```python
from build123d import *

# Parameters (mm, degrees)
F0_W     = 889
F0_H     = 762
F1_DEPTH = 1778
F2_W     = 25.4
F2_H     = 1778
F3_DEPTH = 50.8
F4_W     = 203.0948400497
F4_H     = 157.5736999512
F5_DEPTH = 50.8
F6_SIZE  = 12.7
F7_R     = 38.09999


# Not quite as in the source:
# - a fillet or chamfer is up to 0.001 mm smaller than in the source, because OpenCascade refuses the exact size


with BuildPart() as f1:
    # F0 (on Top) → F1 (new body)
    with BuildSketch(Plane.XY):
        with Locations((444.5, 381)):
            Rectangle(F0_W, F0_H)
    extrude(amount=F1_DEPTH)

    # F2 (on face) → F3 (cut)
    with BuildSketch(Plane.XZ):
        with Locations((431.8, 889)):
            Rectangle(F2_W, F2_H)
    extrude(amount=-F3_DEPTH, mode=Mode.SUBTRACT)

    # F4 (on face) → F5 (cut)
    with BuildSketch(Plane.XZ):
        with Locations((695.2850222588, 1232.5783967972)):
            Rectangle(F4_W, F4_H)
    extrude(amount=-F5_DEPTH, mode=Mode.SUBTRACT)

    # F6
    f6_edges = [f1.edges().sort_by_distance(p)[0] for p in [
        (695.285022, 50.8, 1311.365247),
        (593.737602, 50.8, 1232.578397),
        (695.285022, 50.8, 1153.791547),
        (796.832442, 50.8, 1232.578397),
    ]]
    chamfer(f6_edges, length=F6_SIZE)

    # F7 (radius 38.1 in the source; OpenCascade refuses exactly that, so slightly less here)
    f7_edges = [f1.edges().sort_by_distance(p)[0] for p in [
        (209.55, 0, 0),
        (419.1, 0, 889),
        (209.55, 0, 1778),
        (0, 0, 889),
        (666.75, 0, 0),
        (444.5, 0, 889),
        (889, 0, 889),
        (666.75, 0, 1778),
        (796.832442, 0, 1232.578397),
        (695.285022, 0, 1153.791547),
        (593.737602, 0, 1232.578397),
        (695.285022, 0, 1311.365247),
    ]]
    fillet(f7_edges, radius=F7_R)


solid = f1.part
```
Work out the finished part from the listing and answer in its coordinate system (mm). A direction names the side the tool comes from. Round coordinates to 2 decimals unless told otherwise and drop trailing zeros. Write each question's results on one line, items separated by ' | '.
Q1. Straight lines are drawn through the part: line 1 along X through (y, z) = (34, 98); line 2 along Y through (x, z) = (670.5, 1284.5); line 3 along Z through (x, y) = (397, 36.5). For each, find the intervals that lie inside material, in ascending order. Write a range as [from, to].
Data:
line 1: [0.22, 418.88], [444.72, 888.78] | line 2: [50.8, 762] | line 3: [0.03, 1777.97]
Q2. Determine the mould class of faces 4 (the cylindrical face through (582.873, 11.457, 1234.215)), 5 (the flat face through (664, 0, 877)), 6 (the flat face through (889, 395, 877)) for opening direction X: released by +X, released by -X, zero draft, split by the parting line, or undercut.
Data:
face 4: undercut | face 5: zero draft | face 6: released by +X
Q3. Flat-ended cylindrical pins translate along their axes: P1, Ø7.5, axis at x = 428.5, z = 1155, coming from the -Y side; P2, Ø4, axis at x = 386, z = 1187.5, coming from the -Y side. Find the tip coordinate at first contact, or state that the pin passes through.
Data:
P1: y = 50.8 | P2: y = 0.12
Q4. Which of the six approach directions +Z, -Z, +X, -X, +Y, -Y give full straight-line access (tool end or side, diameter ignored) to faces 1 (the cylindrical face through (877.54, 10.86, 901.45)), 2 (the cylindrical face through (408.24, 11.46, 901.45)), 3 (the cylindrical face through (808.29, 10.865, 1234.215))?
Data:
face 1: +Z, -Z, +X, -Y | face 2: +Z, -Z, -Y | face 3: -Y
